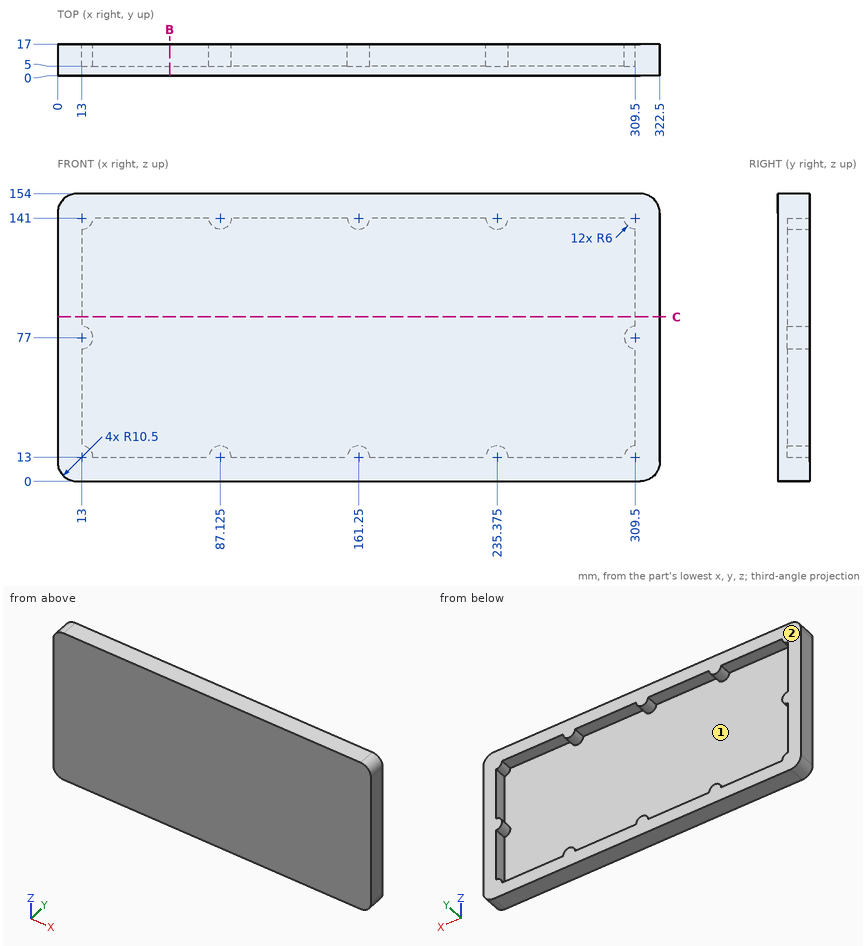
Check sheet for the drawn part. Datum: minimum x, y, z corner. Units: mm. Give positions to 0.01 mm unless a question says otherwise; leave off trailing zeros. Order: outer loops, then holes, each group sorted by start corner. A loop starts at its lowest first (then second) coordinate and runs counter-clockwise, first axis right, second up. Notation, with made-up numbers: (31, 43) -> (68, 43) arc R10 ccw to (68, 53) -> close; hole circle Ø6 at (26.25, 39.5). An arc over 180 degrees is marked (long way). Use a Markdown table: item, result.
1) Mould release check, pull along Z, two halves, no side actions. Record for the marked faces 1 and 2: pulls with the +Z half, pulls with the -Z half, needs draft (parallel to the pull), parting line crosses it, or undercut.
Results:
| item | result |
|---|---|
| face 1 | undercut |
| face 2 | needs draft |
2) Material ranges on probe 1 along X at (y, z) = (8.25, 63.5); probe 2 along Z at (x, y) = (256, 11); probe 3 along X at (y, z) = (9.5, 75.5), recorded low to high.
Results:
| item | result |
|---|---|
| probe 1 | 0 to 13, 309.5 to 322.5 |
| probe 2 | 0 to 13, 141 to 154 |
| probe 3 | 0 to 18.81, 303.69 to 322.5 |
3) Depth check by flat-ended pin: pin 1 Ø6 at (x, z) = (216.5, 30) entering from +Y. Enter the tip coordinate at first touch or a pass-through.
Results:
| item | result |
|---|---|
| pin 1 | y = 5 |
4) Section check B-B, the plane x = 60. Record the boundary of the cut face in (y, z), then the cut area to 3 significant figures.
Results:
| item | result |
|---|---|
| outline | (0, 0) -> (17, 0) -> (17, 13) -> (5, 13) -> (5, 141) -> (17, 141) -> (17, 154) -> (0, 154) -> close |
| area | 1,080 mm² |
5) Section check C-C, the plane z = 88. Record the boundary of the cut face in (x, y).
Results:
| item | result |
|---|---|
| outline | (0, 0) -> (322.5, 0) -> (322.5, 17) -> (309.5, 17) -> (309.5, 5) -> (13, 5) -> (13, 17) -> (0, 17) -> close |
